Source: CAD feature listing. Evaluate the final solid. Frame: model axes, mm. Face numbers are marked on the shaded views. A direction names the side the tool comes from. Round coordinates to 2 decimals unless told otherwise and drop trailing zeros. Write each loop counter-clockwise with the first axis right and the second up, starting at its lowest first coordinate (ties: lowest second). Pieces come first, ordered by that corner, then holes.
from build123d import *

# Parameters (mm, degrees)
SKETCH_1_R                      = 12.55
EXTRUDE_1_DEPTH                 = 8
SKETCH_2_R                      = 3
CUT_EXTRUDE_1_DEPTH             = 7
CUT_EXTRUDE_2_REACH             = 21.468
SKETCH_3_R                      = 1
CUT_EXTRUDE_2_DIRECTION_2_REACH = 21.468
CUT_EXTRUDE_3_DEPTH             = 21
CUT_EXTRUDE_3_DEPTH_BACK        = 19
SKETCH_4_R                      = 1
EXTRUDE_2_DEPTH                 = 2.5
EXTRUDE_2_DEPTH_BACK            = 1
SKETCH_5_R                      = 15
SKETCH_6_R                      = 13.5
CUT_EXTRUDE_4_DEPTH             = 2.5
FILLET_1_R                      = 2
SKETCH_7_W                      = 2.5
SKETCH_7_H                      = 10
CUT_EXTRUDE_5_DEPTH             = 21.5


with BuildPart() as part:
    # 草图1 → 凸台-拉伸1 (new body)
    with BuildSketch(Plane(origin=(0, 0, 0), x_dir=(0, 0, -1), z_dir=(1, 0, 0))):
        Circle(SKETCH_1_R)
    extrude(amount=EXTRUDE_1_DEPTH)

    # 草图2 → 切除-拉伸1 (cut)
    with BuildSketch(Plane.ZY):
        Circle(SKETCH_2_R)
    extrude(amount=-CUT_EXTRUDE_1_DEPTH, mode=Mode.SUBTRACT)

    # 草图3 → 切除-拉伸2 (cut, up to next)
    with BuildSketch(Plane(origin=(0, 0, 0), x_dir=(1, 0, 0), z_dir=(0, 1, 0)), mode=Mode.PRIVATE) as cut_extrude_2_sk1:
        with Locations(Location((2, 0, 0), (0, 0, 270))):
            Circle(SKETCH_3_R)
    cut_extrude_2_tool1 = extrude(cut_extrude_2_sk1.sketch, amount=-CUT_EXTRUDE_2_REACH, mode=Mode.PRIVATE) & part.part
    add(cut_extrude_2_tool1.solids().sort_by_distance((2, 0, 0))[0], mode=Mode.SUBTRACT)

    # 草图3 → 切除-拉伸2 direction 2 (cut, up to next)
    with BuildSketch(Plane(origin=(0, 0, 0), x_dir=(1, 0, 0), z_dir=(0, 1, 0)), mode=Mode.PRIVATE) as cut_extrude_2_direction_2_sk1:
        with Locations(Location((2, 0, 0), (0, 0, 270))):
            Circle(SKETCH_3_R)
    cut_extrude_2_direction_2_tool1 = extrude(cut_extrude_2_direction_2_sk1.sketch, amount=CUT_EXTRUDE_2_DIRECTION_2_REACH, mode=Mode.PRIVATE) & part.part
    add(cut_extrude_2_direction_2_tool1.solids().sort_by_distance((2, 0, 0))[0], mode=Mode.SUBTRACT)

    # 草图4 → 切除-拉伸3 (cut, two sides: drawn at the far end of the back side and taken through both)
    with BuildSketch(Plane.XY.offset(-CUT_EXTRUDE_3_DEPTH_BACK)):
        with Locations(Location((5, 0, 0), (0, 0, 180))):
            Circle(SKETCH_4_R)
    extrude(amount=CUT_EXTRUDE_3_DEPTH + CUT_EXTRUDE_3_DEPTH_BACK, mode=Mode.SUBTRACT)

    # 草图5 → 凸台-拉伸2 (add, two sides: drawn at the far end of the back side and taken through both)
    with BuildSketch(Plane(origin=(8, 0, 0), x_dir=(0, 0, -1), z_dir=(1, 0, 0)).offset(-EXTRUDE_2_DEPTH_BACK)):
        Circle(SKETCH_5_R)
    extrude(amount=EXTRUDE_2_DEPTH + EXTRUDE_2_DEPTH_BACK)

    # 草图6 → 切除-拉伸4 (cut)
    with BuildSketch(Plane(origin=(10.5, 0, 0), x_dir=(0, 0, -1), z_dir=(1, 0, 0))):
        Circle(SKETCH_6_R)
    extrude(amount=-CUT_EXTRUDE_4_DEPTH, mode=Mode.SUBTRACT)

    # 圆角1
    # the kernel refuses this fillet: 2 mm, written as the material it adds along each edge
    with BuildSketch(Plane(origin=(7, 0, 0), x_dir=(0, 0, -1), z_dir=(0, 1, 0))) as fillet_1_piece_1_section:
        with BuildLine():
            CenterArc((12.55 + FILLET_1_R, FILLET_1_R), FILLET_1_R, 180, 90)
            Line((12.55 + FILLET_1_R, 0), (12.55, 0))
            Line((12.55, 0), (12.55, FILLET_1_R))
        make_face()
    fillet_1_piece_1 = revolve(axis=Axis((7, 0, 0), (-1, 0, 0)), mode=Mode.PRIVATE)
    fillet_1_piece_1 = fillet_1_piece_1 - Plane(origin=(5, 0, 13.104940956), x_dir=(-1, 0, 0), z_dir=(0, 0, 1)) * Cylinder(1, 59, mode=Mode.PRIVATE)
    add(fillet_1_piece_1)

    # 草图7 → 切除-拉伸5 (cut)
    with BuildSketch(Plane.XY):
        with Locations((9.25, 0)):
            Rectangle(SKETCH_7_W, SKETCH_7_H)
    extrude(amount=-CUT_EXTRUDE_5_DEPTH, mode=Mode.SUBTRACT)


solid = part.part
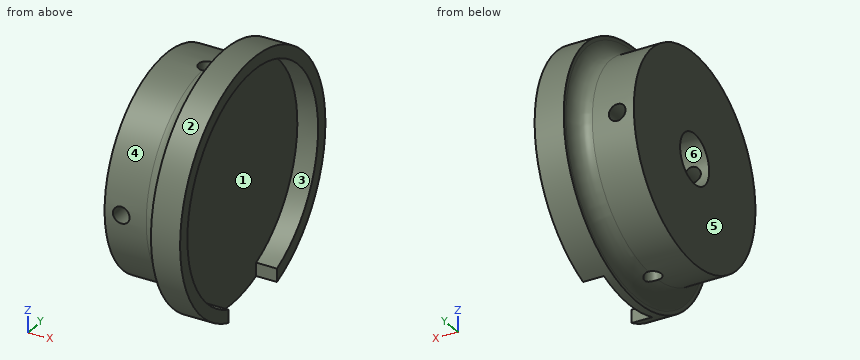
1) Reachability of the marked faces 1 and 2 from +Z, -Z, +X, -X, +Y, -Y: full face, straight path, thin tool, end or side. Return the list, or none.
Taken from the geometry:
face 1: +X
face 2: +X, -X
2) Material intervals for line 1 (X direction, y = 5.25, z = 0); line 2 (X direction, y = 8.5, z = 6.5); line 3 (Z direction, x = 8.6, y = 0), sorted ascending.
Taken from the geometry:
line 1: x = 0 to 1, 3 to 8
line 2: x = 0 to 8
line 3: z = 13.5 to 15
3) Section query D-D on x = 8.75. Return the cut outline in (y, z).
Taken from the geometry:
outline: (-5, -14.14) - (-5, -12.54) arc R13.5 cw (long way) to (5, -12.54) - (5, -14.14) arc R15 ccw (long way) to start
4) Pull-direction query (Z, two-part tool) for the marked faces 3, 4, 5 and 6; classes: released by +Z, released by -Z, zero draft, split by the parting line, or undercut.
Taken from the geometry:
face 3: undercut
face 4: split by the parting line
face 5: zero draft
face 6: undercut
5) Section query C-C on x = 2. Return the cut outline in (y, z), then the cut area to 3 significant figures.
Taken from the geometry:
outline: (-12.51, -1) arc R12.55 ccw to (12.51, -1) - (2.83, -1) arc R3 cw to (-2.83, -1) - close; (-12.51, 1) - (-2.83, 1) arc R3 cw to (2.83, 1) - (12.51, 1) arc R12.55 ccw to start
area: 428 mm2
6) Section query A-A on y = 0. Return the cut outline in (x, z), then the cut area to 3 significant figures.
Taken from the geometry:
outline: (0, -12.55) - (4, -12.55) - (4, -3) - (0, -3) - close; (0, 3) - (4, 3) - (4, 12.55) - (0, 12.55) - close; (6, -12.82) arc R2 cw to (7, -14.55) - (7, -15) - (8, -15) - (8, 13.5) - (10.5, 13.5) - (10.5, 15) - (7, 15) - (7, 14.55) arc R2 cw to (6, 12.82) - (6, 3) - (7, 3) - (7, -3) - (6, -3) - close
area: 131 mm2
7) Contact query for flat-ended pins moving along their axis: P1, Ø1.5, axis at x = 8.5, y = -6.5, coming from the -Z side; P2, Ø1.3, axis at x = 9, z = -13.5, coming from the +Y side; P3, Ø13.5, axis at y = 1, z = 6, coming from the +X side; P4, Ø5, axis at y = 7, z = -1, coming from the -X side. Output: stop coordinate, or through.
Taken from the geometry:
P1: stops at z = -13.85
P2: stops at y = 7.74
P3: stops at x = 8
P4: stops at x = 0
8) Section query B-B on z = 0. Return the cut outline in (x, y), then the cut area to 3 significant figures.
Taken from the geometry:
outline: (0, -12.55) - (1, -12.55) - (1, -3) - (0, -3) - close; (0, 3) - (1, 3) - (1, 12.55) - (0, 12.55) - close; (3, -12.55) - (5, -12.55) arc R2 cw to (7, -14.55) - (7, -15) - (10.5, -15) - (10.5, -13.5) - (8, -13.5) - (8, 13.5) - (10.5, 13.5) - (10.5, 15) - (7, 15) - (7, 14.55) arc R2 cw to (5, 12.55) - (3, 12.55) - (3, 3) - (7, 3) - (7, -3) - (3, -3) - close
area: 135 mm2
